The drawing under review shows one solid part. Ordinate dimensions are in mm from its lowest x, y, z. Coordinates: 2 decimals unless noted, no trailing zeros. Loops run counter-clockwise (first coordinate to the right, second up) from the corner with the lowest first, then second, coordinate; pieces in that order, holes last. Notation, with made-up numbers: M 5.5,50.25 L 33.5,50.25 A21 ccw 33.5,84.25 Z; hole C 34.5,64 d4. An arc over 180 degrees is marked long. Return JSON: item names as keys, results as strings.
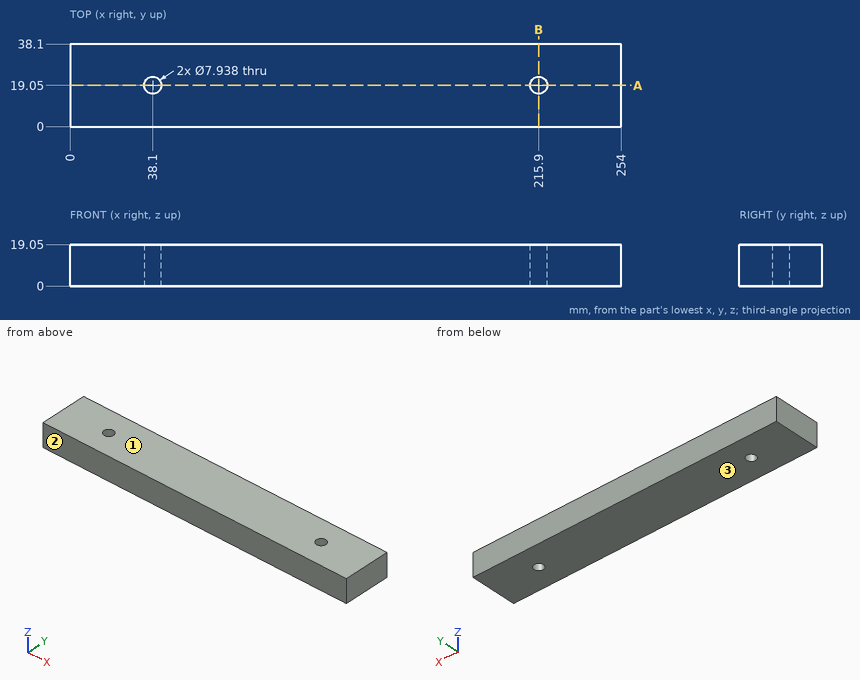
1. To check wall thickness, follow line 1 (X direction, y = 19.05, z = 6.75); line 2 (Y direction, x = 38.1, z = 8.5); line 3 (X direction, y = 15.5, z = 6.5) (1 decimal). State the ranges of each line that lie inside material, in increasing order.
Check values:
{"line 1": "0 to 34.13, 42.07 to 211.93, 219.87 to 254", "line 2": "0 to 15.08, 23.02 to 38.1", "line 3": "0 to 36.3, 39.9 to 214.1, 217.7 to 254"}
2. The part is to be moulded in two halves that separate along Z. For the marked faces 1, 2 and 3, say which applies: released by +Z, released by -Z, zero draft, split by the parting line, or undercut.
Check values:
{"face 1": "released by +Z", "face 2": "zero draft", "face 3": "released by -Z"}
3. Add section B-B on x = 215.9. Give the boundary of the cut face in (y, z).
Check values:
{"outline": "M 0,0 L 15.08,0 L 15.08,19.05 L 0,19.05 Z; M 23.02,0 L 38.1,0 L 38.1,19.05 L 23.02,19.05 Z"}
4. Add section A-A on y = 19.05. Give the boundary of the cut face in (x, z), plus the area to 3 significant figures.
Check values:
{"outline": "M 0,0 L 34.13,0 L 34.13,19.05 L 0,19.05 Z; M 42.07,0 L 211.93,0 L 211.93,19.05 L 42.07,19.05 Z; M 219.87,0 L 254,0 L 254,19.05 L 219.87,19.05 Z", "area": "4,540 mm²"}
